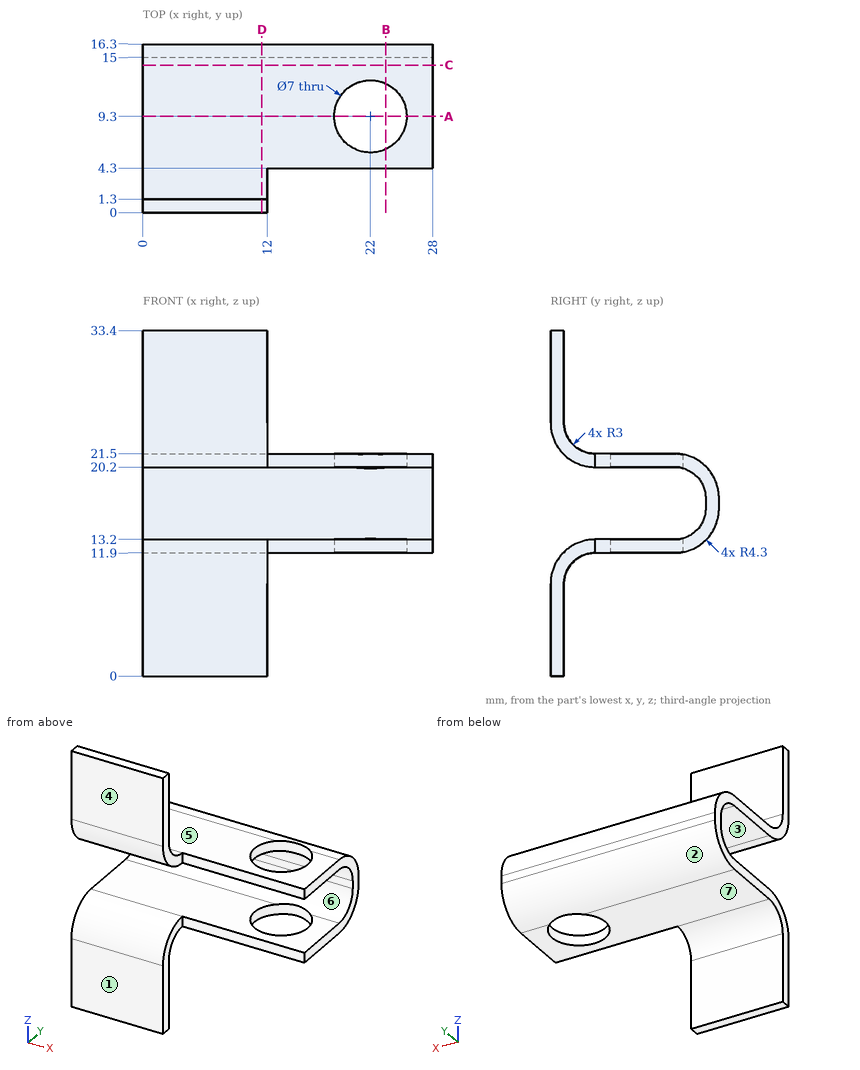
Design review of the part shown in the three views and the two pictorial views. Dimensions are in mm from the part's minimum x, y and z. A direction names the side the tool comes from. Round coordinates to 2 decimals unless told otherwise and drop trailing zeros. Loops run counter-clockwise (first coordinate to the right, second up) from the corner with the lowest first, then second, coordinate; pieces in that order, holes last.
Q1. Machinability: for the marked faces 4, 5, 6 and 7, which of the approach directions +Z, -Z, +X, -X, +Y, -Y give a long, thin tool a straight path to every point of the face, cutting with its end or side? Answer none if there is none.
Result sheet:
face 4: +Z, -Z, +X, -X, -Y
face 5: +Z, +X, -X, +Y
face 6: +X, -X, -Y
face 7: -Z, +X, -X, +Y
Q2. Add section C-C on y = 14.25. Write out the cut boundary in (x, z).
Result sheet:
outline: (0, 12.54) - (28, 12.54) - (28, 14.22) - (0, 14.22) - close; (0, 19.18) - (28, 19.18) - (28, 20.86) - (0, 20.86) - close
Q3. Add section D-D on x = 11.5. Write out the cut boundary in (y, z), plus the area to 3 significant figures.
Result sheet:
outline: (0, 0) - (1.3, 0) - (1.3, 8.9) arc R3 cw to (4.3, 11.9) - (12, 11.9) arc R4.3 ccw to (16.3, 16.2) - (16.3, 17.2) arc R4.3 ccw to (12, 21.5) - (4.3, 21.5) arc R3 cw to (1.3, 24.5) - (1.3, 33.4) - (0, 33.4) - (0, 24.5) arc R4.3 ccw to (4.3, 20.2) - (12, 20.2) arc R3 cw to (15, 17.2) - (15, 16.2) arc R3 cw to (12, 13.2) - (4.3, 13.2) arc R4.3 ccw to (0, 8.9) - close
area: 74.3 mm2
Q4. Add section B-B on x = 23.5. Write out the cut boundary in (y, z), plus the area to 3 significant figures.
Result sheet:
outline: (4.3, 11.9) - (6.14, 11.9) - (6.14, 13.2) - (4.3, 13.2) - close; (4.3, 20.2) - (6.14, 20.2) - (6.14, 21.5) - (4.3, 21.5) - close; (12.46, 11.92) arc R4.3 ccw to (16.3, 16.2) - (16.3, 17.2) arc R4.3 ccw to (12.46, 21.48) - (12.46, 20.16) arc R3 cw to (15, 17.2) - (15, 16.2) arc R3 cw to (12.46, 13.24) - close
area: 19.8 mm2
Q5. To check wall thickness, follow line 1 along X through (y, z) = (9.3, 20.75); line 2 along Z through (x, y) = (25.25, 5.5); line 3 along Y through (x, z) = (22, 21.15). State the ranges of each line that lie inside material, in increasing order.
Result sheet:
line 1: x = 0 to 18.5, 25.5 to 28
line 2: z = 11.9 to 13.2, 20.2 to 21.5
line 3: y = 4.3 to 5.8, 12.8 to 13.7
Q6. Mouldability with a two-part tool opening along Z and no side actions: class the marked faces 1, 2 and 3 as +Z half, -Z half, draft (parallel to the pull), parting line (faces both ways), or undercut.
Result sheet:
face 1: draft
face 2: -Z half
face 3: undercut
Q7. Add section A-A on y = 9.3. Write out the cut boundary in (x, z).
Result sheet:
outline: (0, 11.9) - (18.5, 11.9) - (18.5, 13.2) - (0, 13.2) - close; (0, 20.2) - (18.5, 20.2) - (18.5, 21.5) - (0, 21.5) - close; (25.5, 11.9) - (28, 11.9) - (28, 13.2) - (25.5, 13.2) - close; (25.5, 20.2) - (28, 20.2) - (28, 21.5) - (25.5, 21.5) - close
Q8. Insertion check: pin 1 Ø1.3 at (y, z) = (1.5, 27.5) entering from +X; pin 2 Ø12 at (x, z) = (9, 18) entering from +Y; pin 3 Ø0.7 at (x, z) = (20, 21) entering from -Y; pin 4 Ø1 at (x, y) = (4.5, 6.5) entering from +Z. Each pin has a flat end and moves straight along its axis. Give the tip position at first contact, or say it passes through.
Result sheet:
pin 1: stops at x = 12
pin 2: stops at y = 16.3
pin 3: stops at y = 4.3
pin 4: stops at z = 21.5
